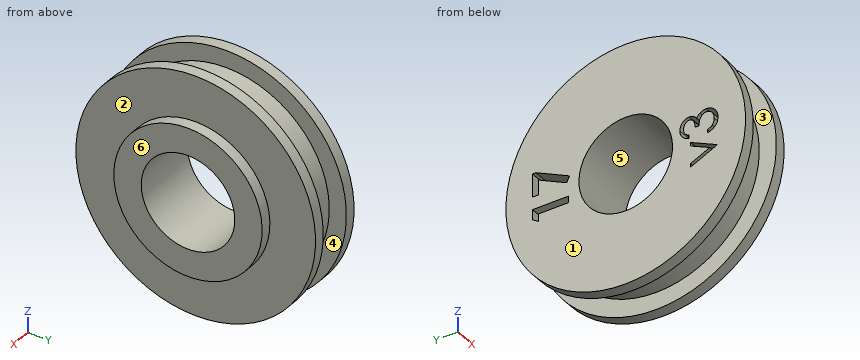
from build123d import *

# Parameters (mm, degrees)
SKETCH1_W           = 5
SKETCH1_H           = 6.4
SKETCH2_W           = 3
SKETCH2_H           = 1.5
SKETCH6_R           = 6.5
SKETCH6_R_2         = 4.1
BOSS_EXTRUDE1_DEPTH = 1
CUT_EXTRUDE2_DEPTH  = 1.5


with BuildPart() as part:
    # Sketch1 → Revolve1 (revolve)
    with BuildSketch(Plane.XY, mode=Mode.PRIVATE) as revolve1_sk:
        with Locations((-3, 7.3)):
            Rectangle(SKETCH1_W, SKETCH1_H)
    revolve(revolve1_sk.sketch.rotate(Axis((0, 0, 0), (1, 0, 0)), 90), axis=Axis((0, 0, 0), (1, 0, 0)))

    # Sketch2 → Cut-Revolve1 (revolve, cut)
    with BuildSketch(Plane.XY, mode=Mode.PRIVATE) as cut_revolve1_sk:
        with Locations((-3, 9.75)):
            Rectangle(SKETCH2_W, SKETCH2_H)
    revolve(cut_revolve1_sk.sketch.rotate(Axis((0, 0, 0), (1, 0, 0)), 90), axis=Axis((0, 0, 0), (1, 0, 0)), mode=Mode.SUBTRACT)

    # Sketch6 → Boss-Extrude1 (add)
    with BuildSketch(Plane(origin=(-0.5, 0, 0), x_dir=(0, 0, -1), z_dir=(1, 0, 0))):
        with Locations(Location((0, 0, 0), (0, 0, 180))):
            Circle(SKETCH6_R)
        with Locations(Location((0, 0, 0), (0, 0, 180))):
            Circle(SKETCH6_R_2, mode=Mode.SUBTRACT)
    extrude(amount=BOSS_EXTRUDE1_DEPTH)

    # Sketch5 → Cut-Extrude2 (cut)
    with BuildSketch(Plane.ZY.offset(5.5)):
        Polygon((-1.793384415, 8.175), (-0.9125, 8.175), (-0.9125, 5), (-1.482371795, 5), (-1.482371795, 7.645833333), (-2.133653846, 7.645833333), align=None)
        Polygon((0.186538462, 8.175), (2.221794872, 8.175), (2.221794872, 7.879251803), (0.821284054, 4.918589744), (0.316286058, 5.172996795), (1.486558494, 7.645833333), (0.186538462, 7.645833333), align=None)
        Polygon((-2.418589744, -5.679807692), (-2.110121194, -5.679807692), (-1.339903846, -7.369070513), (-0.569686498, -5.679807692), (-0.261217949, -5.679807692), (-1.319551282, -8), (-1.36025641, -8), align=None)
        with BuildLine():
            Line((0.430769231, -5.557692308), (0.145833333, -5.557692308))
            add(Edge.make_bspline(
                [(0.145833333, -5.557692308), (0.153552711, -5.525731412), (0.168643464, -5.463250474), (0.20011912, -5.37398103), (0.234408445, -5.289504693), (0.275582847, -5.211403254), (0.320494359, -5.138107107), (0.371949971, -5.071278687), (0.427575719, -5.009218354), (0.489102638, -4.954142774), (0.553626495, -4.90427012), (0.622056471, -4.861747746), (0.693015811, -4.825167979), (0.766996153, -4.795032483), (0.844217751, -4.772330758), (0.923982481, -4.755859941), (1.00649937, -4.745163716), (1.062513256, -4.74411981), (1.090955529, -4.743589744)],
                knots=[0, 0, 0, 0, 1.162005537, 2.271625781, 3.343758855, 4.383309926, 5.390229558, 6.379919256, 7.361854164, 8.333198761, 9.295911338, 10.242430842, 11.177959212, 12.116337295, 13.062827104, 14.020064771, 14.994644689, 16, 16, 16, 16], degree=3))
            add(Edge.make_bspline(
                [(1.090955529, -4.743589744), (1.132396302, -4.744840902), (1.214373905, -4.747315929), (1.334808955, -4.769916882), (1.450947569, -4.805681109), (1.56151853, -4.855096562), (1.664223822, -4.916045053), (1.755605934, -4.988584493), (1.834426226, -5.071315288), (1.90055184, -5.162694114), (1.952327018, -5.26035304), (1.990505371, -5.360864611), (2.013747896, -5.4639904), (2.016760115, -5.533620217), (2.018269231, -5.568504607)],
                knots=[0, 0, 0, 0, 1.083050992, 2.142477498, 3.193116406, 4.255571735, 5.30263384, 6.308962982, 7.297363603, 8.282367274, 9.249857812, 10.179914175, 11.08814088, 12, 12, 12, 12], degree=3))
            add(Edge.make_bspline(
                [(2.018269231, -5.568504607), (2.017213687, -5.602075057), (2.015148153, -5.667767217), (1.99760972, -5.763671718), (1.968094682, -5.854060884), (1.927209968, -5.939315224), (1.874285848, -6.018894186), (1.810175616, -6.092976815), (1.734426773, -6.161891694), (1.677023736, -6.201370073), (1.647470954, -6.221694712)],
                knots=[0, 0, 0, 0, 1.024540389, 2.004866551, 2.965041327, 3.920577974, 4.882998113, 5.874504559, 6.905732034, 8, 8, 8, 8], degree=3))
            add(Edge.make_bspline(
                [(1.647470954, -6.221694712), (1.681245474, -6.238003481), (1.748162567, -6.270315872), (1.839376261, -6.333685023), (1.922178334, -6.406851852), (1.968355279, -6.46394983), (1.99155649, -6.492638221)],
                knots=[0, 0, 0, 0, 1.015518401, 2.012035669, 3.001164323, 4, 4, 4, 4], degree=3))
            add(Edge.make_bspline(
                [(1.99155649, -6.492638221), (2.006833994, -6.513554896), (2.037138821, -6.55504572), (2.074545341, -6.621753764), (2.108480752, -6.689201186), (2.134924165, -6.75919579), (2.155401887, -6.83092631), (2.170039573, -6.904515912), (2.179132901, -6.980024689), (2.180435152, -7.031108153), (2.181089744, -7.056785857)],
                knots=[0, 0, 0, 0, 1.025084078, 2.033381695, 3.024893161, 4.013698104, 4.991890475, 5.976764909, 6.982997093, 8, 8, 8, 8], degree=3))
            add(Edge.make_bspline(
                [(2.181089744, -7.056785857), (2.179461863, -7.101244676), (2.176213764, -7.189953089), (2.147181497, -7.321012301), (2.1021752, -7.449124006), (2.038260694, -7.571656182), (1.960366596, -7.686301242), (1.867695309, -7.788877608), (1.761299782, -7.877050628), (1.642640372, -7.950719906), (1.514082691, -8.009609735), (1.376581975, -8.050483273), (1.232119426, -8.077104287), (1.133052806, -8.079958946), (1.0826873, -8.081410256)],
                knots=[0, 0, 0, 0, 0.955779014, 1.907060117, 2.875433937, 3.871313158, 4.872415639, 5.851225146, 6.836215519, 7.83643374, 8.849228613, 9.86973379, 10.916971861, 12, 12, 12, 12], degree=3))
            add(Edge.make_bspline(
                [(1.0826873, -8.081410256), (1.048742649, -8.080622663), (0.981950895, -8.079072942), (0.883758578, -8.068478782), (0.790031037, -8.04912942), (0.700641545, -8.023091422), (0.61551069, -7.990078913), (0.534898252, -7.94896838), (0.458308277, -7.900607231), (0.386463514, -7.844424619), (0.319372528, -7.781576547), (0.258818271, -7.710947302), (0.203791173, -7.633842514), (0.155764636, -7.549366599), (0.112551115, -7.458611259), (0.07700839, -7.360414407), (0.045725053, -7.255653901), (0.03118041, -7.182649094), (0.023717949, -7.145192308)],
                knots=[0, 0, 0, 0, 1.048658725, 2.063410685, 3.046034179, 4.001477787, 4.936774919, 5.862367409, 6.792675028, 7.730719943, 8.675894397, 9.627829632, 10.600096036, 11.597688215, 12.626045268, 13.701542398, 14.82072376, 16, 16, 16, 16], degree=3))
            Line((0.023717949, -7.145192308), (0.308653846, -7.145192308))
            add(Edge.make_bspline(
                [(0.308653846, -7.145192308), (0.316077261, -7.169638913), (0.330516446, -7.217189683), (0.355094845, -7.285624817), (0.383096778, -7.348361051), (0.413136413, -7.405858597), (0.444685432, -7.458683705), (0.479986828, -7.505439544), (0.516425981, -7.548179763), (0.543893681, -7.572259518), (0.557336739, -7.584044471)],
                knots=[0, 0, 0, 0, 1.198163088, 2.33053128, 3.407730985, 4.417276592, 5.372219308, 6.28897303, 7.162600585, 8, 8, 8, 8], degree=3))
            add(Edge.make_bspline(
                [(0.557336739, -7.584044471), (0.575113633, -7.597749888), (0.610612549, -7.625118417), (0.668459444, -7.660044894), (0.729296877, -7.69030811), (0.794443045, -7.713425463), (0.862492159, -7.732999484), (0.934544126, -7.745808812), (1.009963272, -7.754597367), (1.061459744, -7.755372912), (1.087775441, -7.755769231)],
                knots=[0, 0, 0, 0, 0.946170439, 1.889420265, 2.845303464, 3.807233317, 4.801018734, 5.828864929, 6.890507805, 8, 8, 8, 8], degree=3))
            add(Edge.make_bspline(
                [(1.087775441, -7.755769231), (1.117487547, -7.755210517), (1.175587005, -7.754118), (1.260363913, -7.744070751), (1.341015669, -7.729438162), (1.416646823, -7.706838528), (1.488248069, -7.678915898), (1.554815708, -7.643856273), (1.617223605, -7.602722133), (1.674672423, -7.555968753), (1.726330133, -7.504786397), (1.771813834, -7.451253111), (1.810480491, -7.395594608), (1.841671309, -7.337502884), (1.866300737, -7.277218498), (1.88306764, -7.214572274), (1.8947258, -7.150076897), (1.895675227, -7.106235618), (1.896153846, -7.084134615)],
                knots=[0, 0, 0, 0, 1.217147791, 2.380027433, 3.494444702, 4.572153297, 5.609568379, 6.639424714, 7.649109417, 8.668170816, 9.669597737, 10.625200337, 11.543417969, 12.441394052, 13.322311151, 14.205496177, 15.095365482, 16, 16, 16, 16], degree=3))
            add(Edge.make_bspline(
                [(1.896153846, -7.084134615), (1.894765644, -7.054551472), (1.891996147, -6.995532388), (1.870851936, -6.908702874), (1.836073109, -6.825043064), (1.787384474, -6.745980312), (1.728115634, -6.672705029), (1.658841755, -6.607325899), (1.578987576, -6.553378031), (1.505490981, -6.516104749), (1.440389731, -6.490671117), (1.384677204, -6.473730256), (1.322305142, -6.459385012), (1.254027812, -6.44603888), (1.179330751, -6.434680228), (1.098295282, -6.425208009), (1.010904984, -6.417628794), (0.95040657, -6.414244157), (0.919230769, -6.4125)],
                knots=[0, 0, 0, 0, 1.07054697, 2.135767047, 3.216561865, 4.33974944, 5.486079747, 6.621378074, 7.775625952, 8.963672916, 9.598146892, 10.304877434, 11.070270905, 11.915000392, 12.823868403, 13.805723172, 14.86925407, 16, 16, 16, 16], degree=3))
            Line((0.919230769, -6.4125), (0.919230769, -6.086858974))
            add(Edge.make_bspline(
                [(0.919230769, -6.086858974), (0.958511112, -6.086192402), (1.035451655, -6.084886752), (1.147841489, -6.069095199), (1.255313708, -6.04725063), (1.355486538, -6.013790491), (1.446789299, -5.974928222), (1.526000653, -5.929705146), (1.592010851, -5.879436052), (1.644499108, -5.823345042), (1.683986337, -5.76318782), (1.712857789, -5.700489138), (1.729912371, -5.634699454), (1.732188997, -5.58980072), (1.733333333, -5.567232572)],
                knots=[0, 0, 0, 0, 1.321986639, 2.589447074, 3.816329219, 5.01088745, 6.139805852, 7.153945165, 8.075214402, 8.924034688, 9.728124013, 10.488707548, 11.240355623, 12, 12, 12, 12], degree=3))
            add(Edge.make_bspline(
                [(1.733333333, -5.567232572), (1.732957403, -5.550652046), (1.732209509, -5.517665876), (1.722777692, -5.46947385), (1.708604455, -5.422755134), (1.689119272, -5.377708406), (1.663038735, -5.334646087), (1.63182759, -5.293201044), (1.59466367, -5.253609901), (1.552077443, -5.21670704), (1.506346735, -5.181537803), (1.456227296, -5.151680433), (1.403230309, -5.126148841), (1.347297101, -5.105094507), (1.288246156, -5.089256438), (1.226354921, -5.077884639), (1.16150538, -5.070774766), (1.117262451, -5.069751132), (1.094771635, -5.069230769)],
                knots=[0, 0, 0, 0, 0.884392785, 1.759457502, 2.611959086, 3.489218968, 4.37281399, 5.2945488, 6.255912374, 7.266815255, 8.301784654, 9.332968512, 10.37626691, 11.440494194, 12.520033166, 13.637162961, 14.798855837, 16, 16, 16, 16], degree=3))
            add(Edge.make_bspline(
                [(1.094771635, -5.069230769), (1.058620479, -5.070492933), (0.988008863, -5.072958233), (0.886213903, -5.094550967), (0.791581364, -5.129002514), (0.719247002, -5.170126039), (0.665832095, -5.210721075), (0.627662302, -5.246174383), (0.590178696, -5.285574159), (0.55584726, -5.331347113), (0.521127296, -5.380393416), (0.489518301, -5.435206327), (0.458802723, -5.494356028), (0.440294695, -5.536171353), (0.430769231, -5.557692308)],
                knots=[0, 0, 0, 0, 1.472543308, 2.876219568, 4.221790263, 5.565193594, 6.249813518, 6.953379497, 7.687249741, 8.463570142, 9.283606569, 10.136032583, 11.040678096, 12, 12, 12, 12], degree=3))
        make_face()
    extrude(amount=-CUT_EXTRUDE2_DEPTH, mode=Mode.SUBTRACT)


solid = part.part
Work out the finished part from the listing and answer in its coordinate system (mm). Face numbers are marked on the shaded views. A direction names the side the tool comes from. Round coordinates to 2 decimals unless told otherwise and drop trailing zeros. Write each loop counter-clockwise with the first axis right and the second up, starting at its lowest first coordinate (ties: lowest second). Pieces come first, ordered by that corner, then holes.
1) A tool of negligible diameter and unlimited length cuts with its end or side. For the marked faces 1, 2 and 3, from which of +Z, -Z, +X, -X, +Y, -Y can it reach the whole face along a straight path? Write none if from no direction.
2) Given pin 1 Ø3 at (x, z) = (-1, 2) entering from -Y; pin 2 Ø0.6 at (x, y) = (-5, 8) entering from +Z; pin 3 Ø1.2 at (x, y) = (-5, 6) entering from +Z (3 decimals); pin 4 Ø5 at (y, z) = (0, 0) entering from -X, each flat-ended and moving along its own axis, determine where each tip first touches the part or whether it passes through.
3) A cutting plane is placed at A-A (y = 0). Give the vertices of the cut face in (x, z).
4) The mould has two halves that part along X. Classify the marked faces 4, 5 and 6: pulls with the +X half, pulls with the -X half, needs draft (parallel to the pull), parting line crosses it, or undercut.
5) Straight lines are drawn through the part: line 1 (Y direction, x = -3.1, z = 0); line 2 (X direction, y = 4.25, z = 9); line 3 (Y direction, x = -1.05, z = 0). For each, find the intervals that lie inside material, in ascending order.
6) A cutting plane is placed at C-C (x = 0). Give the vertices of the cut face in (y, z).
7) A cutting plane is placed at D-D (x = -3.5). Give the vertices of the cut face in (y, z).
8) A cutting plane is placed at B-B (z = -3.5). Give the vertices of the cut face in (x, y).
Completed:
1. face 1: +Z, -Z, -X, +Y, -Y
1. face 2: +X
1. face 3: none
2. pin 1: stops at y = -10.49
2. pin 2: stops at z = 7.14
2. pin 3: stops at z = 9.005
2. pin 4: passes through
3. outline: (-5.5, -10.5) - (-4.5, -10.5) - (-4.5, -9) - (-1.5, -9) - (-1.5, -10.5) - (-0.5, -10.5) - (-0.5, -6.5) - (0.5, -6.5) - (0.5, -4.1) - (-5.5, -4.1) - close; (-5.5, 4.1) - (0.5, 4.1) - (0.5, 6.5) - (-0.5, 6.5) - (-0.5, 10.5) - (-1.5, 10.5) - (-1.5, 9) - (-4.5, 9) - (-4.5, 10.5) - (-5.5, 10.5) - close
4. face 4: undercut
4. face 5: needs draft
4. face 6: pulls with the +X half
5. line 1: y = -9 to -4.1, 4.1 to 9
5. line 2: x = -5.5 to -4.5, -1.5 to -0.5
5. line 3: y = -10.5 to -4.1, 4.1 to 10.5
6. outline: circle Ø13 at (0, 0); hole circle Ø8.2 at (0, 0)
7. outline: circle Ø18 at (0, 0); hole circle Ø8.2 at (0, 0)
8. outline: (-5.5, -9.9) - (-4.5, -9.9) - (-4.5, -8.29) - (-1.5, -8.29) - (-1.5, -9.9) - (-0.5, -9.9) - (-0.5, -5.48) - (0.5, -5.48) - (0.5, -2.14) - (-5.5, -2.14) - close; (-5.5, 2.14) - (0.5, 2.14) - (0.5, 5.48) - (-0.5, 5.48) - (-0.5, 9.9) - (-1.5, 9.9) - (-1.5, 8.29) - (-4.5, 8.29) - (-4.5, 9.9) - (-5.5, 9.9) - close
